Check sheet for the modelled part. Datum: model origin and axes. Units: mm. A direction names the side the tool comes from. Coordinates: 2 decimals unless noted, no trailing zeros. Loops run counter-clockwise (first coordinate to the right, second up) from the corner with the lowest first, then second, coordinate; pieces in that order, holes last. Notation, with made-up numbers: M 32,85 L 61,85 A23 cw 61,112 Z; hole C -18.5,20 d10. An arc over 180 degrees is marked long. Answer as CSV lines item,"result". Start each with the question number.
from build123d import *

# Parameters (mm, degrees)
F0_W     = 128.30928
F0_H     = 25.661856
F1_DEPTH = 203.454
F2_R     = 20.542437
F3_DEPTH = 25.4


with BuildPart() as f1:
    # F0 (on Front) → F1 (new body)
    with BuildSketch(Plane.XZ):
        with Locations((-1.558043, 12.830928)):
            Rectangle(F0_W, F0_H)
    extrude(amount=-F1_DEPTH)

    # F2 (on face) → F3 (join)
    with BuildSketch(Plane(origin=(-65.712683, 0, 0), x_dir=(0, -1, 0), z_dir=(-1, 0, 0))):
        with Locations((-190.771684, 13.703045)):
            Circle(F2_R)
    extrude(amount=F3_DEPTH)


solid = f1.part
Item 1: Set-up check for faces 1 (the face through (-78.235, 171.178, 19.873)), 2 (the face through (-2, 0, 13)), 3 (the face through (-2, 203.454, 13)): record each of +Z, -Z, +X, -X, +Y, -Y from which the full face is reachable in a straight line by a thin tool's end or side.
Item 2: Sectioned sample at B-B, the plane x = 39.5. Record the boundary of the cut face in (y, z).
Item 3: Go/stop test with flat-tipped pins: pin 1 (8 mm diameter, centred on x = 11, y = 112, fed in from +Z); pin 2 (6 mm diameter, centred on x = 40.5, z = 10.5, fed in from +Y); pin 3 (2 mm diameter, centred on y = 101.5, z = 7.5, fed in from -X). Record where each tip stops, or that it passes through.
Item 4: Material ranges on line 1 (X direction, y = 122.5, z = 12); line 2 (Y direction, x = 16, z = 2); line 3 (Z direction, x = 25, y = 75), recorded low to high. Write a range as from..to.
Item 5: Sectioned sample at D-D, the plane z = 4. Record the boundary of the cut face in (x, y).
Item 6: Sectioned sample at A-A, the plane z = 22. Record the boundary of the cut face in (x, y), and give its area (3 significant figures).
Item 7: Sectioned sample at C-C, the plane y = 76.5. Record the boundary of the cut face in (x, z).
Reply:
1,face 1,"-X"
1,face 2,"+Z, -Z, +X, -X, -Y"
1,face 3,"+Z, -Z, +X, +Y"
2,outline,"M 0,0 L 203.45,0 L 203.45,25.66 L 0,25.66 Z"
3,pin 1,"z = 25.66"
3,pin 2,"y = 203.45"
3,pin 3,"x = -65.71"
4,line 1,"-65.71..62.6"
4,line 2,"0..203.45"
4,line 3,"0..25.66"
5,outline,"M -91.11,172.67 L -65.71,172.67 L -65.71,0 L 62.6,0 L 62.6,203.45 L -65.71,203.45 L -65.71,208.88 L -91.11,208.88 Z"
6,outline,"M -91.11,171.98 L -65.71,171.98 L -65.71,0 L 62.6,0 L 62.6,203.45 L -65.71,203.45 L -65.71,209.56 L -91.11,209.56 Z"
6,area,"27,100 mm²"
7,outline,"M -65.71,0 L 62.6,0 L 62.6,25.66 L -65.71,25.66 Z"
